Here's how the part is built. I have some questions about the finished solid (model axes, mm). Face numbers are marked on the shaded views. Round coordinates to 2 decimals unless told otherwise and drop trailing zeros. Order: outer loops, then holes, each group sorted by start corner. A loop starts at its lowest first (then second) coordinate and runs counter-clockwise, first axis right, second up. Notation, with made-up numbers: M 68,27 L 75,27 A15 ccw 75,42 Z; hole C 71.25,88 d5. An arc over 180 degrees is marked long. Answer as CSV lines item,"result". Start each with the question number.
Autodesk Inventor part; units mm, degrees
ref_plane "YZ Plane" through (0, 0, 0) normal (1, 0, 0) x (0, 1, 0)
ref_plane "XZ Plane" through (0, 0, 0) normal (0, 1, 0) x (-1, 0, 0)
ref_plane "XY Plane" through (0, 0, 0) normal (0, 0, 1) x (1, 0, 0)
sketch "Sketch1" plane through (0, 0, 0) normal (0, 0, 1) x (1, 0, 0)
  line L0 (60, -25) -> (-60, -25)
  line L1 (-60, -25) -> (-60, 25)
  line L2 (-60, 25) -> (60, 25)
  line L3 (60, 25) -> (60, -25)
  line L4 (60, -25) -> (-60, 25) construction
  line L5 (-60, -25) -> (60, 25) construction
  line L6 (50, -13.5) -> (-21.5, -13.5)
  line L7 (-21.5, -13.5) -> (-21.5, 13.5)
  line L8 (-21.5, 13.5) -> (50, 13.5)
  line L9 (50, 13.5) -> (50, -13.5)
  line L10 (50, -13.5) -> (-21.5, 13.5) construction
  line L11 (-21.5, -13.5) -> (50, 13.5) construction
  line L12 (-33.5, -13.1) -> (-52.2, -13.1)
  line L13 (-52.2, -13.1) -> (-52.2, 13.1)
  line L14 (-52.2, 13.1) -> (-33.5, 13.1)
  line L15 (-33.5, 13.1) -> (-33.5, -13.1)
  line L16 (-33.5, -13.1) -> (-52.2, 13.1) construction
  line L17 (-52.2, -13.1) -> (-33.5, 13.1) construction
  circle A0 centre (-41.9, 0) radius 3.5
  line L18 (-5, 28) -> (5, 28)
  line L19 (5, 28) -> (5, 25)
  line L20 (5, 25) -> (-5, 25)
  line L21 (-5, 25) -> (-5, 28)
  line L22 (-5, -25) -> (5, -25)
  line L23 (5, -25) -> (5, -28)
  line L24 (5, -28) -> (-5, -28)
  line L25 (-5, -28) -> (-5, -25)
  line L26 (-60, 28) -> (-50, 28)
  line L27 (-50, 28) -> (-50, 25)
  line L28 (-50, 25) -> (-60, 25)
  line L29 (-60, 25) -> (-60, 28)
  line L30 (50, 28) -> (60, 28)
  line L31 (60, 28) -> (60, 25)
  line L32 (60, 25) -> (50, 25)
  line L33 (50, 25) -> (50, 28)
  line L34 (-60, -25) -> (-50, -25)
  line L35 (-50, -25) -> (-50, -28)
  line L36 (-50, -28) -> (-60, -28)
  line L37 (-60, -28) -> (-60, -25)
  line L38 (50, -25) -> (60, -25)
  line L39 (60, -25) -> (60, -28)
  line L40 (60, -28) -> (50, -28)
  line L41 (50, -28) -> (50, -25)
  line L42 (-63, 5) -> (-60, 5)
  line L43 (-60, 5) -> (-60, -5)
  line L44 (-60, -5) -> (-63, -5)
  line L45 (-63, -5) -> (-63, 5)
  line L46 (63, -5) -> (60, -5)
  line L47 (60, -5) -> (60, 5)
  line L48 (60, 5) -> (63, 5)
  line L49 (63, 5) -> (63, -5)
  point P0 (0, 0)
  point P1 (14.25, 0)
  point P2 (-42.85, 0)
  point P3 (0, 25)
  point P4 (0, -25)
  point P5 (-60, 0)
  point P6 (60, 0)
  dimension "d0" = 120
  dimension "d1" = 50
  dimension "d2" = 27
  dimension "d3" = 71.5
  dimension "d4" = 10
  dimension "d6" = 18.7
  dimension "d7" = 26.2
  dimension "d8" = 7
  dimension "d9" = 8.4
  dimension "d10" = 12
  dimension "d11" = 10
  dimension "d12" = 3
  dimension "d13" = 10
  dimension "d14" = 3
  dimension "d15" = 10
  dimension "d16" = 3
  dimension "d17" = 10
  dimension "d18" = 3
  dimension "d19" = 10
  dimension "d20" = 3
  dimension "d21" = 10
  dimension "d22" = 3
  dimension "d23" = 3
  dimension "d24" = 10
  dimension "d25" = 3
  dimension "d26" = 10
extrude "Extrusion1" add sketch "Sketch1" along normal blind 3 contours L39 L40 L41 L0 | L0 L1 L2 L3 | L3 L48 L49 L46 | L23 L24 L25 L0 | L2 L33 L30 L31 | L35 L36 L37 L0 | L2 L21 L18 L19 | L44 L45 L42 L1 | L2 L29 L26 L27 | L12 L13 L14 L15
sketch "Sketch2" plane through (0, 0, 3) normal (0, 0, 1) x (1, 0, 0)
  line L0 (-60, 28) -> (-60, 5)
  line L1 (-50, 28) -> (-60, 28)
  line L2 (-50, 25) -> (-50, 28)
  line L3 (-5, 25) -> (-50, 25)
  line L4 (60, 5) -> (60, 28)
  line L5 (60, 28) -> (50, 28)
  line L6 (50, 28) -> (50, 25)
  line L7 (50, 25) -> (5, 25)
  line L8 (5, 25) -> (5, 28)
  line L9 (5, 28) -> (-5, 28)
  line L10 (-5, 28) -> (-5, 25)
  line L11 (-60, 25) -> (60, 25)
  point P0 (0, 0)
extrude "Extrusion2" cut sketch "Sketch2" against normal through all
sketch "Sketch3" plane through (0, 0, 3) normal (0, 0, 1) x (1, 0, 0)
  line L0 (60, 25) -> (-60, 25)
  line L1 (-35, 28) -> (-25, 28)
  line L2 (-25, 28) -> (-25, 25)
  line L3 (-25, 25) -> (-35, 25)
  line L4 (-35, 25) -> (-35, 28)
  line L5 (25, 28) -> (35, 28)
  line L6 (35, 28) -> (35, 25)
  line L7 (35, 25) -> (25, 25)
  line L8 (25, 25) -> (25, 28)
  point P0 (0, 0)
  point P1 (-30, 25)
  point P2 (0, 25)
  point P3 (-30, 28)
  point P4 (30, 25)
  dimension "d31" = 120
  dimension "d32" = 10
  dimension "d33" = 3
  dimension "d34" = 10
  dimension "d35" = 3
  dimension "d36" = 30
  dimension "d37" = 30
extrude "Extrusion3" add sketch "Sketch3" against normal blind 3
sketch "Sketch4" plane through (0, 0, 3) normal (0, 0, 1) x (1, 0, 0)
  circle A0 centre (-41.9, 0) radius 3.5
  line L0 (50, -13.5) -> (50, 13.5)
  line L1 (50, 13.5) -> (-21.5, 13.5)
  line L2 (-21.5, 13.5) -> (-21.5, -13.5)
  line L3 (-21.5, -13.5) -> (50, -13.5)
  line L4 (60, 5) -> (63, 5)
  line L5 (63, 5) -> (63, -5)
  line L6 (63, -5) -> (60, -5)
  line L7 (60, -5) -> (60, -28)
  line L8 (60, -28) -> (50, -28)
  line L9 (50, -28) -> (50, -25)
  line L10 (50, -25) -> (5, -25)
  line L11 (5, -25) -> (5, -28)
  line L12 (5, -28) -> (-5, -28)
  line L13 (-5, -28) -> (-5, -25)
  line L14 (-5, -25) -> (-50, -25)
  line L15 (-50, -25) -> (-50, -28)
  line L16 (-50, -28) -> (-60, -28)
  line L17 (-60, -28) -> (-60, -5)
  line L18 (-60, -5) -> (-63, -5)
  line L19 (-63, -5) -> (-63, 5)
  line L20 (-63, 5) -> (-60, 5)
  line L21 (-60, 5) -> (-60, 25)
  line L22 (-60, 25) -> (-35, 25)
  line L23 (-35, 25) -> (-35, 28)
  line L24 (-35, 28) -> (-25, 28)
  line L25 (-25, 28) -> (-25, 25)
  line L26 (-25, 25) -> (25, 25)
  line L27 (25, 25) -> (25, 28)
  line L28 (25, 28) -> (35, 28)
  line L29 (35, 28) -> (35, 25)
  line L30 (35, 25) -> (60, 25)
  line L31 (60, 25) -> (60, 5)
  point P0 (0, 0)
properties part number "Front-panel"
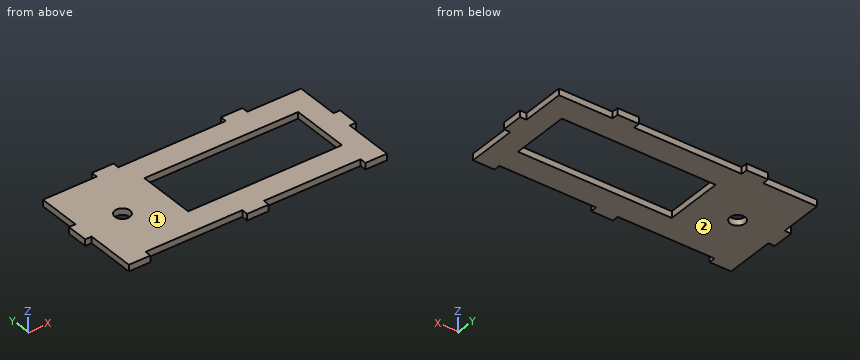
Item 1: We'd pull the mould along Z, two halves only. Please class the marked faces 1 and 2: pulls with the +Z half, pulls with the -Z half, needs draft (parallel to the pull), parting line crosses it, or undercut.
Item 2: For P1, Ø0.9, axis at x = 62, z = 1.5, coming from the +Y side; P2, Ø1.5, axis at y = -27, z = 2, coming from the -X side; P3, Ø1.5, axis at y = 26.5, z = 2, coming from the +X side, each with a flat end and sliding along its axis, tell me the tip position at first contact or that it passes through.
Item 3: If we section it at D-D on y = 0: Please give me the cut outline in (x, z), and give its area (4 significant figures).
Item 4: If we section it at A-A on x = 30: Please give me the cut outline in (y, z), and give its area (3 significant figures).
Item 5: If we section it at B-B on y = -12: Please give me the cut outline in (x, z), and give its area (4 significant figures).
Item 6: If we section it at C-C on z = 1.75: Count the separate pieces of the cut face and the enclosed holes in it, and give its area (3 significant figures).
Item 7: If I drill on line 1 along Y through (x, z) = (-41.9, 0.7); line 2 along Y through (x, z) = (-14.5, 0.7); line 3 along X through (y, z) = (10, 0.9), over which ranges is the centre line in solid material (lowest first)?
Geometry says:
1,face 1,"pulls with the +Z half"
1,face 2,"pulls with the -Z half"
2,P1,"y = 5"
2,P2,"x = -60"
2,P3,"x = 35"
3,outline,"M -63,0 L -45.4,0 L -45.4,3 L -63,3 Z; M -38.4,0 L -21.5,0 L -21.5,3 L -38.4,3 Z; M 50,0 L 63,0 L 63,3 L 50,3 Z"
3,area,"142.5 mm²"
4,outline,"M -25,0 L -13.5,0 L -13.5,3 L -25,3 Z; M 13.5,0 L 28,0 L 28,3 L 13.5,3 Z"
4,area,"78.0 mm²"
5,outline,"M -60,0 L -21.5,0 L -21.5,3 L -60,3 Z; M 50,0 L 60,0 L 60,3 L 50,3 Z"
5,area,"145.5 mm²"
6,separate pieces,"1"
6,enclosed holes,"2"
6,area,"4,240 mm²"
7,line 1,"-25 to -3.5, 3.5 to 25"
7,line 2,"-25 to -13.5, 13.5 to 25"
7,line 3,"-60 to -21.5, 50 to 60"
